Here's how the part is built. I have some questions about the finished solid (model axes, mm). A direction names the side the tool comes from. Round coordinates to 2 decimals unless told otherwise and drop trailing zeros. Loops run counter-clockwise (first coordinate to the right, second up) from the corner with the lowest first, then second, coordinate; pieces in that order, holes last. Notation, with made-up numbers: M 15,-6.75 L 35,-6.75 A27 cw 35,27.25 Z; hole C 82.25,24.5 d1. An arc over 180 degrees is marked long. Put each result on its own line as item: value. Start each with the question number.
```python
from build123d import *

# Parameters (mm, degrees)
SKETCH1_R           = 17
BOSS_EXTRUDE1_DEPTH = 5
SKETCH2_R           = 3
BOSS_EXTRUDE2_DEPTH = 30
SKETCH3_R           = 3.125
BOSS_EXTRUDE3_DEPTH = 4
FILLET1_R           = 3


with BuildPart() as part:
    # Sketch1 → Boss-Extrude1 (new body)
    with BuildSketch(Plane.XY):
        Circle(SKETCH1_R)
    extrude(amount=BOSS_EXTRUDE1_DEPTH)

    # Sketch2 → Boss-Extrude2 (add)
    with BuildSketch(Plane.XY.offset(5)):
        with Locations((-9.768207719, 0)):
            Circle(SKETCH2_R)
        with Locations((9.768207719, 0)):
            Circle(SKETCH2_R)
    extrude(amount=BOSS_EXTRUDE2_DEPTH)

    # Sketch3 → Boss-Extrude3 (add)
    with BuildSketch(Plane(origin=(0, 0, 0), x_dir=(-1, 0, 0), z_dir=(0, 0, -1))):
        Circle(SKETCH3_R)
    extrude(amount=BOSS_EXTRUDE3_DEPTH)

    # Fillet1
    fillet1_edges = [part.edges().sort_by_distance(p)[0] for p in [
        (-12.768207719, 0, 35),
        (6.768207719, 0, 35),
    ]]
    fillet(fillet1_edges, radius=FILLET1_R)


solid = part.part
```
1) If we mould it in two halves opening along X, with no side actions, what happens to faces 4 (the face through (7.39, -1.83, 18.31)), 5 (the face through (4, 0, 0)), 6 (the face through (9.139, 14.334, 2.465))? For each: pulls with the +X half, pulls with the -X half, needs draft (parallel to the pull), parting line crosses it, or undercut.
2) On a 3-axis mill with a long thin cutter (end or side, diameter ignored), from which of +Z, -Z, +X, -X, +Y, -Y can I reach the whole of each face in a straight line? I mean faces 1 (the face through (0, 0, -4)), 2 (the face through (-2.98, 0.94, -1.97)), 3 (the face through (-12.765, 0.132, 18.311)). Say none if no direction works.
3) I'm going to push flat-ended pins straight in: P1, Ø10, axis at x = 9.5, z = 18, coming from the -Y side; P2, Ø10, axis at x = 9, z = 27.5, coming from the +Y side; P3, Ø6, axis at x = -2, y = 3.5, coming from the +Z side. Where does each tip first touch, or does it pass through?
4) Suppose I cut it at C-C (z = 10). Write out the boundary of the cut face in (x, y).
5) If I drill on probe 1 along Z at (x, y) = (2.5, 7); probe 2 along X at (y, z) = (-1, 17); probe 3 along X at (y, z) = (-0.5, 23), over which ranges is the centre line in solid material (lowest first)? Write a range as from..to.
6) Suppose I cut it at B-B (y = 0). Write out the boundary of the cut face in (x, z) (3 decimals), plus the area to 3 significant figures.
7) Suppose I cut it at D-D (x = 10.5). Write out the boundary of the cut face in (y, z).
8) Suppose I cut it at A-A (x = 0). Write out the boundary of the cut face in (y, z) (3 decimals).
Results are:
1. face 4: undercut
1. face 5: needs draft
1. face 6: parting line crosses it
2. face 1: -Z, +X, -X, +Y, -Y
2. face 2: -Z
2. face 3: +Z
3. P1: y = -3
3. P2: y = 3
3. P3: z = 5
4. outline: C -9.77,0 d6; C 9.77,0 d6
5. probe 1: 0..5
5. probe 2: -12.6..-6.94, 6.94..12.6
5. probe 3: -12.73..-6.81, 6.81..12.73
6. outline: M -17,0 L -3.125,0 L -3.125,-4 L 3.125,-4 L 3.125,0 L 17,0 L 17,5 L 12.768,5 L 12.768,32 A3 ccw 6.768,32 L 6.768,5 L -6.768,5 L -6.768,32 A3 ccw -12.768,32 L -12.768,5 L -17,5 Z
6. area: 547 mm²
7. outline: M -13.37,0 L 13.37,0 L 13.37,5 L 2.91,5 L 2.91,32 A2.91 ccw -2.91,32 L -2.91,5 L -13.37,5 Z
8. outline: M -17,0 L -3.125,0 L -3.125,-4 L 3.125,-4 L 3.125,0 L 17,0 L 17,5 L -17,5 Z
